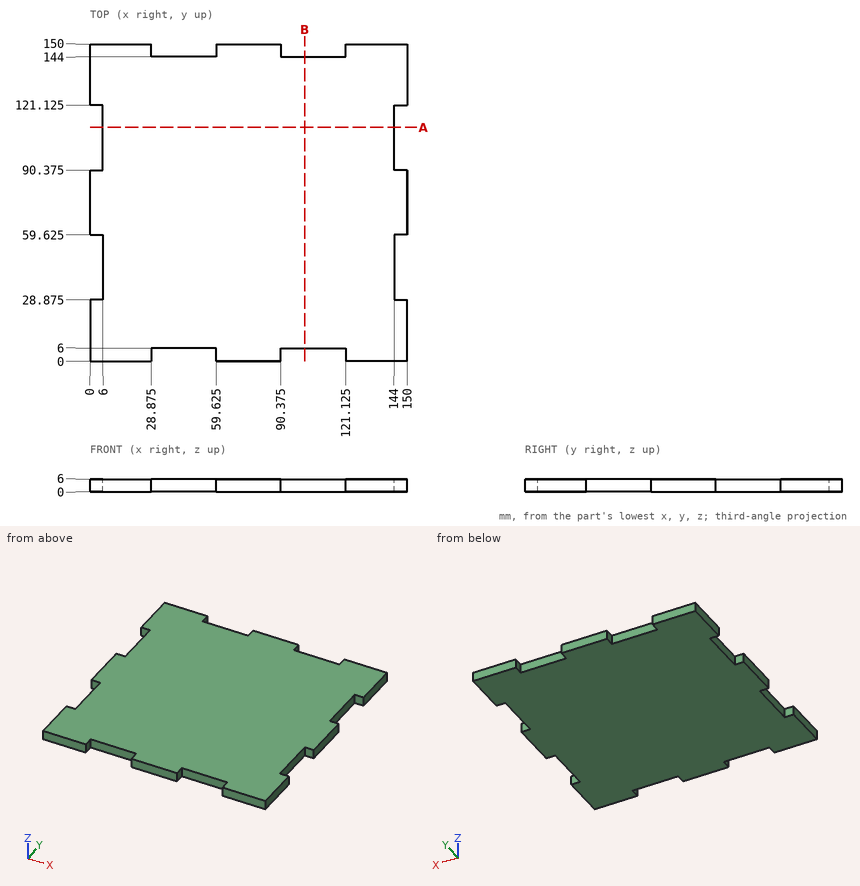
Design review of the part shown in the three views and the two pictorial views. Dimensions are in mm from the part's minimum x, y and z. Round coordinates to 2 decimals unless told otherwise and drop trailing zeros. Write each loop counter-clockwise with the first axis right and the second up, starting at its lowest first coordinate (ties: lowest second). Pieces come first, ordered by that corner, then holes. Notation, with made-up numbers: (-7, 27.5) - (47, 27.5) arc R13 ccw to (47, 36.5) - close; hole circle Ø3 at (73, 86). An arc over 180 degrees is marked (long way). Return JSON: item names as keys, results as strings. Group by question number.
Item 1: We need section A-A on y = 110.5. Write out the cut boundary in (x, z), and give its area (3 significant figures).
Item 2: For probe 1 along Y at (x, z) = (39, 4.8), list the stretches that pass through material, from the lowest coordinate up. Write a range as [from, to].
Item 3: Insertion check: P1, Ø1.8, axis at x = 47.5, z = 4, coming from the -Y side; P2, Ø3, axis at y = 99.5, z = 4.5, coming from the +X side. Each pin has a flat end and moves straight along its axis. Give the tip position at first contact, or say it passes through.
Model answer:
{
 "1": {"outline": "(6, 0) - (144, 0) - (144, 6) - (6, 6) - close", "area": "828 mm²"},
 "2": {"probe 1": "y = [6, 144]"},
 "3": {"P1": "stops at y = 6", "P2": "stops at x = 144"}
}
